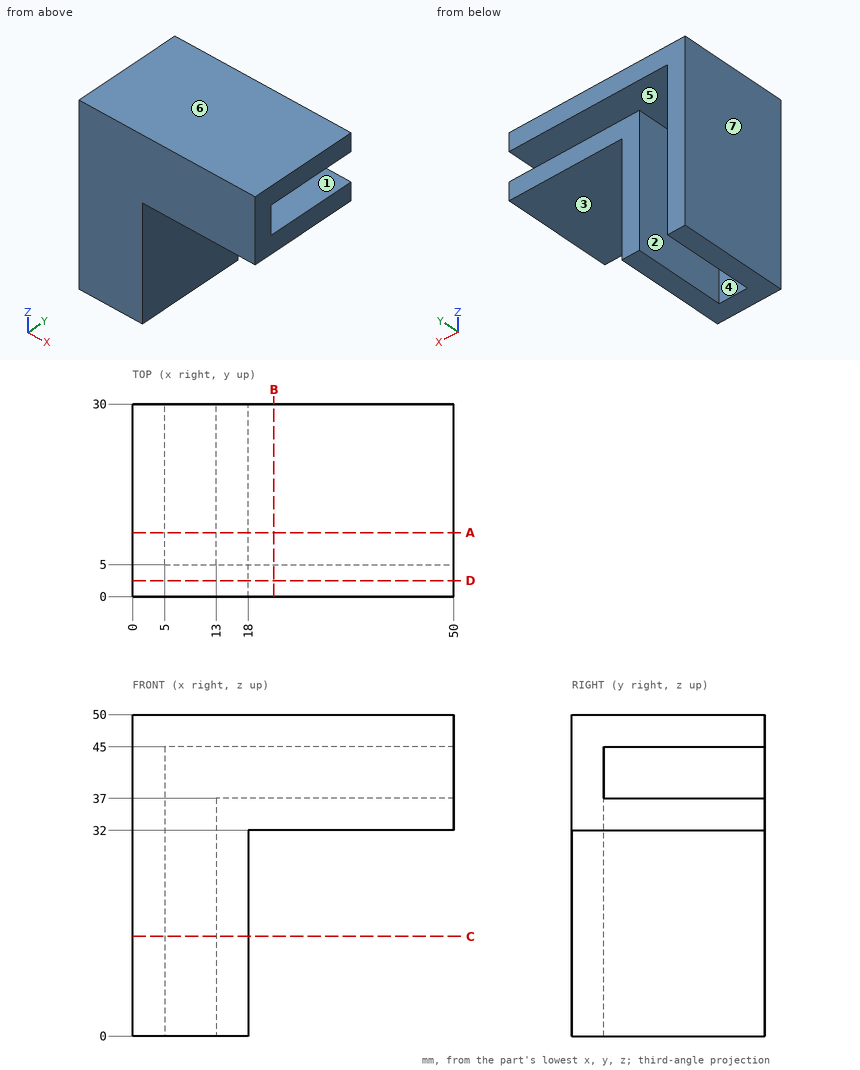
Study the drawing (mm; zero at the part's minimum x, y, z) and answer. A direction names the side the tool comes from. Give positions to 0.01 mm unless a question says otherwise; leave off trailing zeros. Order: outer loops, then holes, each group sorted by start corner. A loop starts at its lowest first (then second) coordinate and runs counter-clockwise, first axis right, second up. Notation, with made-up numbers: (10, 72.25) - (60, 72.25) arc R26 ccw to (60, 92.25) - close; hole circle Ø1 at (-21.75, 34.25). An arc over 180 degrees is marked (long way). Answer in a Markdown table with one row per item. Add a question column.
Q1. The part is cut by section B-B (x = 22). Determine the outline of the cut face in (y, z), then the cut area to 3 significant figures.
Q2. The part is cut by section A-A (y = 10). Determine the outline of the cut face in (x, z).
Q3. Find the intervals of material crossed by line 1 along Z through (x, y) = (44, 8); line 2 along X through (y, z) = (24, 10.5); line 3 along Z through (x, y) = (16, 21.5), in increasing order. Write a range as [from, to].
Q4. For a pull along Z with two mould halves and no side action, classify the marked faces 4, 5, 6 and 7 as released by +Z, released by -Z, zero draft, split by the parting line, or undercut.
Q5. Which of the six approach directions +Z, -Z, +X, -X, +Y, -Y give full straight-line access (tool end or side, diameter ignored) to the marked faces 1, 2 and 3?
Q6. The part is cut by section D-D (y = 2.5). Determine the outline of the cut face in (x, z).
Q7. Given P1, Ø15, axis at y = 13.5, z = 14, coming from the +X side; P2, Ø2, axis at x = 7, z = 7.5, coming from the +Y side; P3, Ø12.5, axis at x = 29.5, y = 16, coming from the -Z side, each flat-ended and moving along its own axis, determine where each tip first touches the part or whether it passes through.
Q8. The part is cut by section C-C (z = 15.5). Determine the outline of the cut face in (x, y).
Determined:
| question | item | result |
|---|---|---|
| 1 | outline | (0, 32) - (30, 32) - (30, 37) - (5, 37) - (5, 45) - (30, 45) - (30, 50) - (0, 50) - close |
| 1 | area | 340 mm² |
| 2 | outline | (0, 0) - (5, 0) - (5, 45) - (50, 45) - (50, 50) - (0, 50) - close; (13, 0) - (18, 0) - (18, 32) - (50, 32) - (50, 37) - (13, 37) - close |
| 3 | line 1 | z = [32, 37], [45, 50] |
| 3 | line 2 | x = [0, 5], [13, 18] |
| 3 | line 3 | z = [0, 37], [45, 50] |
| 4 | face 4 | undercut |
| 4 | face 5 | undercut |
| 4 | face 6 | released by +Z |
| 4 | face 7 | zero draft |
| 5 | face 1 | +X, +Y |
| 5 | face 2 | -Z, +Y |
| 5 | face 3 | -Z, +X, +Y, -Y |
| 6 | outline | (0, 0) - (18, 0) - (18, 32) - (50, 32) - (50, 50) - (0, 50) - close |
| 7 | P1 | stops at x = 18 |
| 7 | P2 | stops at y = 5 |
| 7 | P3 | stops at z = 32 |
| 8 | outline | (0, 0) - (18, 0) - (18, 30) - (13, 30) - (13, 5) - (5, 5) - (5, 30) - (0, 30) - close |
